Could you check a few things on this model? Use its own coordinates, in mm. Coordinates: 2 decimals unless noted, no trailing zeros. Loops run counter-clockwise (first coordinate to the right, second up) from the corner with the lowest first, then second, coordinate; pieces in that order, holes last.
from build123d import *

# Parameters (mm, degrees)
SKETCH_1_W      = 75
SKETCH_1_H      = 20
SKETCH_1_R      = 2.1
EXTRUDE_1_DEPTH = 3


with BuildPart() as part:
    # 草图1 → 凸台-拉伸1 (new body)
    with BuildSketch(Plane(origin=(36, 0, 0), x_dir=(0, -1, 0), z_dir=(-1, 0, 0))):
        with Locations((42.5, 10)):
            Rectangle(SKETCH_1_W, SKETCH_1_H)
        with Locations(Location((20, 15, 0), (0, 0, 270))):
            Circle(SKETCH_1_R, mode=Mode.SUBTRACT)
        with Locations(Location((55, 10, 0), (0, 0, 270))):
            Circle(SKETCH_1_R, mode=Mode.SUBTRACT)
        with Locations(Location((45, 10, 0), (0, 0, 270))):
            Circle(SKETCH_1_R, mode=Mode.SUBTRACT)
        with Locations(Location((35, 10, 0), (0, 0, 270))):
            Circle(SKETCH_1_R, mode=Mode.SUBTRACT)
        with Locations(Location((20, 5, 0), (0, 0, 270))):
            Circle(SKETCH_1_R, mode=Mode.SUBTRACT)
        with Locations(Location((75, 5, 0), (0, 0, 270))):
            Circle(SKETCH_1_R, mode=Mode.SUBTRACT)
        with Locations(Location((70, 15, 0), (0, 0, 270))):
            Circle(SKETCH_1_R, mode=Mode.SUBTRACT)
        with Locations(Location((65, 5, 0), (0, 0, 270))):
            Circle(SKETCH_1_R, mode=Mode.SUBTRACT)
    extrude(amount=-EXTRUDE_1_DEPTH)


solid = part.part
(1) Imagine slicing it at C-C, the plane y = -45. Write out the boundary of the cut face in (x, z).
Answers:
outline: (36, 0) - (39, 0) - (39, 7.9) - (36, 7.9) - close; (36, 12.1) - (39, 12.1) - (39, 20) - (36, 20) - close
(2) Imagine slicing it at A-A, the plane y = -20. Write out the boundary of the cut face in (x, z).
Answers:
outline: (36, 0) - (39, 0) - (39, 2.9) - (36, 2.9) - close; (36, 7.1) - (39, 7.1) - (39, 12.9) - (36, 12.9) - close; (36, 17.1) - (39, 17.1) - (39, 20) - (36, 20) - close
(3) Imagine slicing it at D-D, the plane x = 37.4. State how many separate pieces and enclosed holes the cut face has, and give its area (3 significant figures).
Answers:
separate pieces: 1
enclosed holes: 8
area: 1,390 mm2
(4) For pin 1 (2.5 mm diameter, centred on y = -65, z = 5, fed in from -X), with a flat end and sliding along its axis, tell me the tip position at first contact or that it passes through.
Answers:
pin 1: passes through
(5) I need wall thicknesses on probe 1 along Y at (x, z) = (37.8, 10); probe 2 along Y at (x, z) = (37.2, 5); probe 3 along Z at (x, y) = (36.85, -20). Which ranges of each line are inside material? Lowest first, please.
Answers:
probe 1: y = -80 to -57.1, -52.9 to -47.1, -42.9 to -37.1, -32.9 to -5
probe 2: y = -80 to -77.1, -72.9 to -67.1, -62.9 to -22.1, -17.9 to -5
probe 3: z = 0 to 2.9, 7.1 to 12.9, 17.1 to 20
(6) We'd pull the mould along Z, two halves only. Please class faces 1 (the face through (36, -42, 10)), 2 (the face through (37.479, -68.722, 16.666)), 3 (the face through (37, -42, 0)), 4 (the face through (37, -42, 20)): +Z half, -Z half, draft (parallel to the pull), parting line (faces both ways), or undercut.
Answers:
face 1: draft
face 2: undercut
face 3: -Z half
face 4: +Z half
(7) Imagine slicing it at B-B, the plane z = 5. Write out the boundary of the cut face in (x, y).
Answers:
outline: (36, -80) - (39, -80) - (39, -77.1) - (36, -77.1) - close; (36, -72.9) - (39, -72.9) - (39, -67.1) - (36, -67.1) - close; (36, -62.9) - (39, -62.9) - (39, -22.1) - (36, -22.1) - close; (36, -17.9) - (39, -17.9) - (39, -5) - (36, -5) - close
